Here's the drawing with two shaded views (mm, measured from the low corner). I have some questions. A direction names the side the tool comes from. Round coordinates to 2 decimals unless told otherwise and drop trailing zeros. Loops run counter-clockwise (first coordinate to the right, second up) from the corner with the lowest first, then second, coordinate; pieces in that order, holes last. Notation, with made-up numbers: (71, 39.25) - (117, 39.25) arc R31 cw to (117, 65.25) - close; hole circle Ø5 at (-39.75, 53.25). An arc over 180 degrees is marked (long way). Answer as CSV lines item,"result".
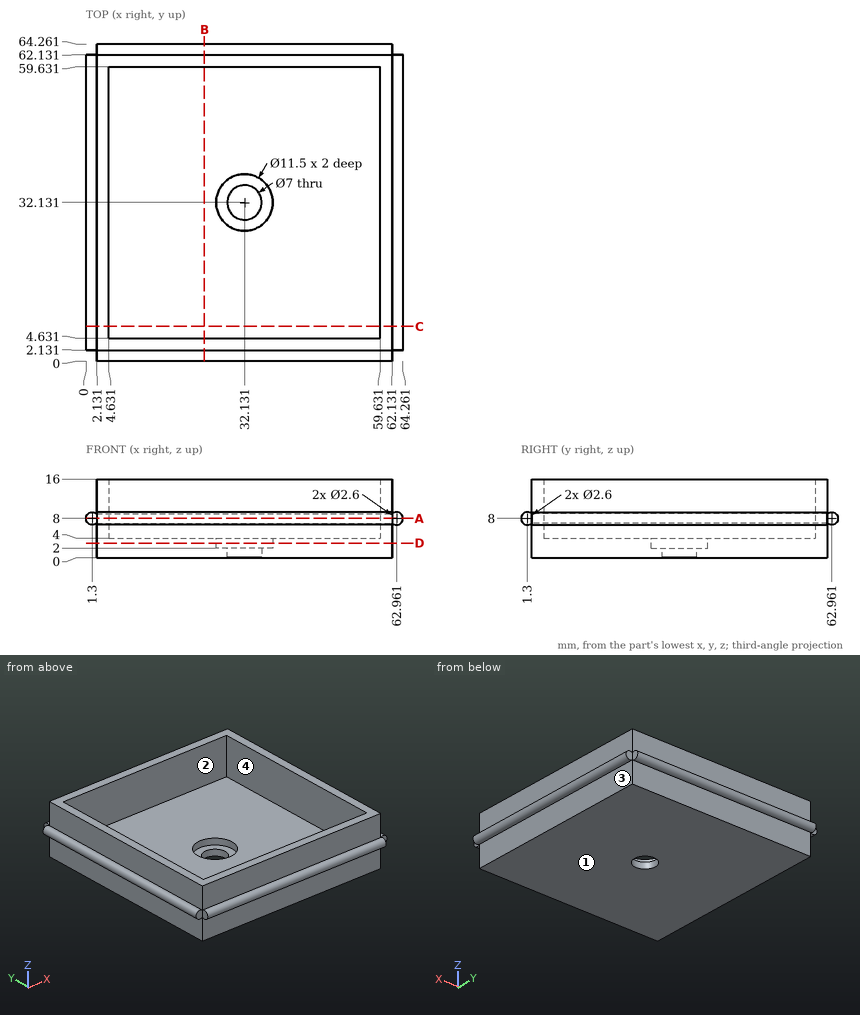
Q1. On a 3-axis mill with a long thin cutter (end or side, diameter ignored), from which of +Z, -Z, +X, -X, +Y, -Y can I reach the whole of each face in a straight line? I mean the marked faces 1 and 2. Say none if no direction works.
Checks:
face 1,"-Z, +X, -X, +Y, -Y"
face 2,"+Z"
Q2. I'm going to push flat-ended pins straight in: pin 1 Ø0.6 at (x, z) = (0.5, 7.5) entering from +Y; pin 2 Ø2 at (y, z) = (22, 12) entering from -X; pin 3 Ø1.7 at (x, z) = (1.5, 7.5) entering from -Y; pin 4 Ø5 at (y, z) = (16, 5) entering from +X. Where does each tip first touch, or does it pass through?
Checks:
pin 1,"y = 62.13"
pin 2,"x = 2.13"
pin 3,"y = 0"
pin 4,"x = 64.16"
Q3. Imagine slicing it at B-B (x = 24). Write out the boundary of the cut face in (y, z), then the cut area to 3 significant figures.
Checks:
outline,"(2.13, 0) - (62.13, 0) - (62.13, 7) arc R1.3 ccw (long way) to (62.13, 9) - (62.13, 16) - (59.63, 16) - (59.63, 4) - (4.63, 4) - (4.63, 16) - (2.13, 16) - (2.13, 9) arc R1.3 ccw (long way) to (2.13, 7) - close"
area,"309 mm²"
Q4. If I drill on line 1 along X through (y, z) = (31.5, 12.75); line 2 along X through (y, z) = (42.5, 8), over which ranges is the centre line in solid material (lowest first)? Write a range as [from, to].
Checks:
line 1,"[2.13, 4.63], [59.63, 62.13]"
line 2,"[0, 4.63], [59.63, 64.26]"
Q5. We'd pull the mould along Y, two halves only. Please class the marked faces 3 and 4: pulls with the +Y half, pulls with the -Y half, needs draft (parallel to the pull), parting line crosses it, or undercut.
Checks:
face 3,"needs draft"
face 4,"undercut"
Q6. Imagine slicing it at D-D (z = 3). Write out the boundary of the cut face in (x, y).
Checks:
outline,"(2.13, 2.13) - (62.13, 2.13) - (62.13, 62.13) - (2.13, 62.13) - close; hole circle Ø11.5 at (32.13, 32.13)"
Q7. Imagine slicing it at A-A (z = 8). Write out the boundary of the cut face in (x, y), then the cut area to 3 significant figures.
Checks:
outline,"(0, 2.13) - (2.13, 2.13) - (2.13, 0) - (62.13, 0) - (62.13, 2.13) - (64.26, 2.13) - (64.26, 62.13) - (62.13, 62.13) - (62.13, 64.26) - (2.13, 64.26) - (2.13, 62.13) - (0, 62.13) - close; hole (4.63, 4.63) - (59.63, 4.63) - (59.63, 59.63) - (4.63, 59.63) - close"
area,"1,090 mm²"
